from build123d import *

# Parameters (mm, degrees)
BOSS_EXTRUDE1_DEPTH     = 100
SKETCH2_R               = 3
CUT_EXTRUDE1_DEPTH      = 6
CUT_EXTRUDE1_DEPTH_BACK = 6


with BuildPart() as part:
    # Sketch1 → Boss-Extrude1 (new body, symmetric)
    with BuildSketch(Plane(origin=(0, 0, 0), x_dir=(0, 0, -1), z_dir=(1, 0, 0))):
        Polygon((0, 5.773502692), (-5, 2.886751346), (-5, -2.886751346), (0, -5.773502692), (5, -2.886751346), (5, 2.886751346), align=None)
    extrude(amount=BOSS_EXTRUDE1_DEPTH, both=True)

    # Sketch2 → Cut-Extrude1 (cut, two sides)
    with BuildSketch(Plane.XY) as cut_extrude1_sk:
        with Locations((90, 0)):
            Circle(SKETCH2_R)
        with Locations((-90, 0)):
            Circle(SKETCH2_R)
    extrude(amount=CUT_EXTRUDE1_DEPTH, mode=Mode.SUBTRACT)
    extrude(cut_extrude1_sk.sketch, amount=-CUT_EXTRUDE1_DEPTH_BACK, mode=Mode.SUBTRACT)


solid = part.part
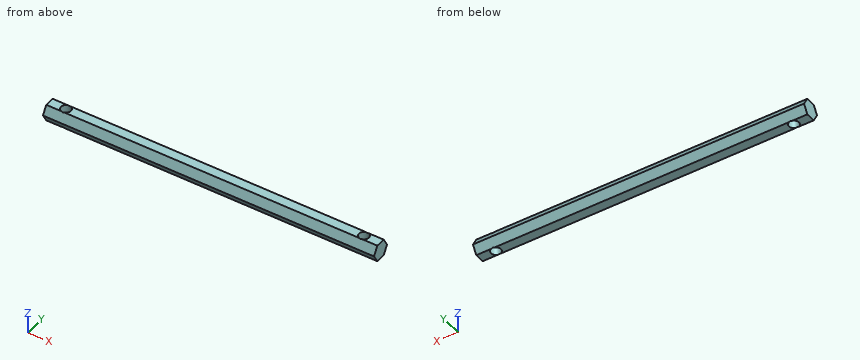
Input: part model. Units: mm. Frame: model coordinates. Coordinates: 2 decimals unless noted, no trailing zeros. Write each loop counter-clockwise with the first axis right and the second up, starting at its lowest first coordinate (ties: lowest second). Pieces come first, ordered by that corner, then holes. Notation, with made-up numbers: M 67,64.25 L 86,64.25 A16 cw 86,71.25 Z; hole C -5.75,78 d6. An arc over 180 degrees is marked long. Answer as a JSON object with one key per item and string values. Group by question number.
(1) Section B-B on x = -58.5. Output: boundary loops of the cut face in (y, z).
(2) Section A-A on y = 0. Output: boundary loops of the cut face in (x, z).
(3) Contact query for flat-ended pins moving along their axis: P1, Ø1, axis at x = 5, z = 2, coming from the +Y side; P2, Ø2, axis at x = 5, z = 3.5, coming from the -Y side. Output: stop coordinate, or through.
(4) Section C-C on z = 2. Output: boundary loops of the cut face in (x, y).
(5) Ray query, line 1 along X through (y, z) = (0, 1.55); line 2 along X through (y, z) = (2.25, -4.25); line 3 along Y through (x, z) = (-90, -1.7). Return the intervals inside material, ascending. Write a range as [from, to].
Result set:
{
 "1": {"outline": "M -5.77,0 L -2.89,-5 L 2.89,-5 L 5.77,0 L 2.89,5 L -2.89,5 Z"},
 "2": {"outline": "M -100,-5 L -93,-5 L -93,5 L -100,5 Z; M -87,-5 L 87,-5 L 87,5 L -87,5 Z; M 93,-5 L 100,-5 L 100,5 L 93,5 Z"},
 "3": {"P1": "stops at y = 4.91", "P2": "stops at y = -4.33"},
 "4": {"outline": "M -100,-4.62 L 100,-4.62 L 100,4.62 L -100,4.62 Z; hole C -90,0 d6; hole C 90,0 d6"},
 "5": {"line 1": "x = [-100, -93], [-87, 87], [93, 100]", "line 2": "x = [-100, -91.98], [-88.02, 88.02], [91.98, 100]", "line 3": "y = [-4.79, -3], [3, 4.79]"}
}
